The figure shows three views and two pictorial views of one solid part (mm, origin at its lowest corner). Answer the questions. Give positions to 0.01 mm unless a question says otherwise; leave off trailing zeros. Write each loop counter-clockwise with the first axis right and the second up, starting at its lowest first coordinate (ties: lowest second). Pieces come first, ordered by that corner, then holes. Notation, with made-up numbers: M 63.25,-25 L 101.25,-25 A26 ccw 101.25,6 Z; hole C 68.25,28.5 d5. An arc over 180 degrees is marked long. Return JSON: item names as keys, results as strings.
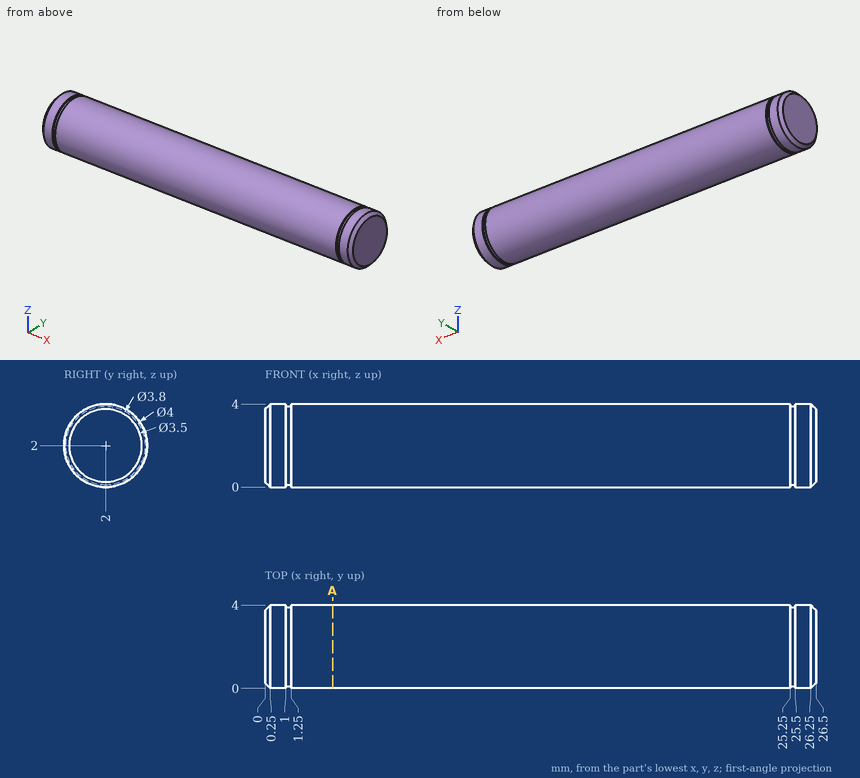
Item 1: Given pin 1 Ø1 at (x, z) = (18, 2.5) entering from +Y, flat-ended and moving along its own axis, determine where the tip first touches the part or whether it passes through.
Geometry results:
{"pin 1": "stops at y = 4"}
Item 2: Find the intervals of material crossed by line 1 (Y direction, x = 19, z = 2.1); line 2 (X direction, y = 1, z = 3.7); line 3 (Z direction, x = 19.25, y = 1.3), in increasing order.
Geometry results:
{"line 1": "y = 0 to 4", "line 2": "x = 0.22 to 1, 1.25 to 25.25, 25.5 to 26.28", "line 3": "z = 0.13 to 3.87"}
Item 3: A cutting plane is placed at A-A, the plane x = 3.25. Write down the section's boundary in (y, z), plus the area to 3 significant figures.
Geometry results:
{"outline": "C 2,2 d4", "area": "12.6 mm2"}
